Could you check a few things on this model? Use its own coordinates, in mm. Coordinates: 2 decimals unless noted, no trailing zeros. Write each loop counter-clockwise with the first axis right and the second up, starting at its lowest first coordinate (ties: lowest second). Pieces come first, ordered by that corner, then holes.
Item 1: If I drill on probe 1 along X at (y, z) = (66.5, 1.55); probe 2 along X at (y, z) = (56.5, 1.8); probe 3 along Y at (x, z) = (39, 1.8), over which ranges is the centre line in solid material (lowest first)?
Item 2: I want a section at A-A on x = 0. Please give me the cut outline in (y, z).
Item 3: I want a section at B-B on y = -71.5. Please give me the cut outline in (x, z), then the cut area to 3 significant figures.
Item 4: I want a section at D-D on y = 71.5. Please give me the cut outline in (x, z).
Item 5: I want a section at C-C on z = 1.2. State how many separate pieces and enclosed holes the cut face has, then the cut area to 3 significant figures.
Item 6: For P1, Ø1, axis at y = -6, z = 1, coming from the +X side, with a flat end and sliding along its axis, tell me the tip position at first contact or that it passes through.
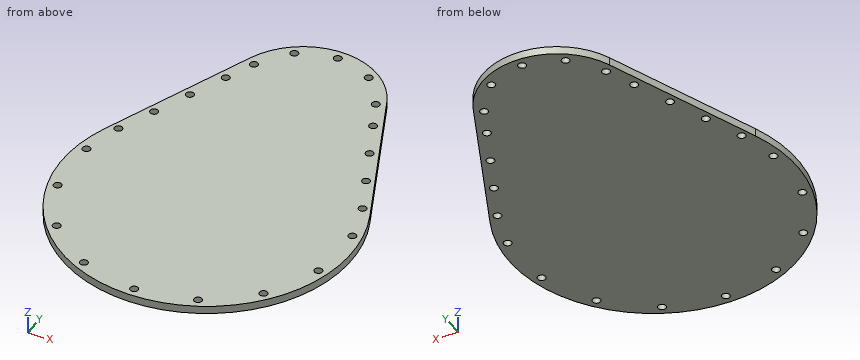
from build123d import *

# Parameters (mm, degrees)
SKETCH1_R           = 1.5
BOSS_EXTRUDE1_DEPTH = 3


with BuildPart() as part:
    # Sketch1 → Boss-Extrude1 (new body)
    with BuildSketch(Plane.XY):
        with BuildLine():
            Line((-25.751949598, 57.992592593), (-50.124330467, 0.896296296))
            ThreePointArc((-50.124330467, 0.896296296), (0, -75), (50.124330467, 0.896296296))
            Line((50.124330467, 0.896296296), (25.751949598, 57.992592593))
            ThreePointArc((25.751949598, 57.992592593), (0, 75), (-25.751949598, 57.992592593))
        make_face()
        with Locations((0, -71.5)):
            Circle(SKETCH1_R, mode=Mode.SUBTRACT)
        with Locations((0, 71.5)):
            Circle(SKETCH1_R, mode=Mode.SUBTRACT)
        with Locations((14.052622691, 67.069225085)):
            Circle(SKETCH1_R, mode=Mode.SUBTRACT)
        with Locations((23.022469209, 55.379493511)):
            Circle(SKETCH1_R, mode=Mode.SUBTRACT)
        with Locations((21.553531349, -66.721697139)):
            Circle(SKETCH1_R, mode=Mode.SUBTRACT)
        with Locations((39.068266599, -53.282168094)):
            Circle(SKETCH1_R, mode=Mode.SUBTRACT)
        with Locations((49.262217141, -33.6997713)):
            Circle(SKETCH1_R, mode=Mode.SUBTRACT)
        with Locations((50.225195404, -11.643942939)):
            Circle(SKETCH1_R, mode=Mode.SUBTRACT)
        with Locations((27.835315177, 44.555939465)):
            Circle(SKETCH1_R, mode=Mode.SUBTRACT)
        with Locations((33.935175216, 30.757307943)):
            Circle(SKETCH1_R, mode=Mode.SUBTRACT)
        with Locations((40.035035255, 16.95867642)):
            Circle(SKETCH1_R, mode=Mode.SUBTRACT)
        with Locations((46.134895294, 3.160044897)):
            Circle(SKETCH1_R, mode=Mode.SUBTRACT)
        with Locations((-46.134895294, 3.160044897)):
            Circle(SKETCH1_R, mode=Mode.SUBTRACT)
        with Locations((-40.035035255, 16.95867642)):
            Circle(SKETCH1_R, mode=Mode.SUBTRACT)
        with Locations((-33.935175216, 30.757307943)):
            Circle(SKETCH1_R, mode=Mode.SUBTRACT)
        with Locations((-27.835315177, 44.555939465)):
            Circle(SKETCH1_R, mode=Mode.SUBTRACT)
        with Locations((-50.225195404, -11.643942939)):
            Circle(SKETCH1_R, mode=Mode.SUBTRACT)
        with Locations((-49.262217141, -33.6997713)):
            Circle(SKETCH1_R, mode=Mode.SUBTRACT)
        with Locations((-39.068266599, -53.282168094)):
            Circle(SKETCH1_R, mode=Mode.SUBTRACT)
        with Locations((-21.553531349, -66.721697139)):
            Circle(SKETCH1_R, mode=Mode.SUBTRACT)
        with Locations((-23.022469209, 55.379493511)):
            Circle(SKETCH1_R, mode=Mode.SUBTRACT)
        with Locations((-14.052622691, 67.069225085)):
            Circle(SKETCH1_R, mode=Mode.SUBTRACT)
    extrude(amount=BOSS_EXTRUDE1_DEPTH)


solid = part.part
Response values:
1. probe 1: x = -20.09 to -15.44, -12.66 to 12.66, 15.44 to 20.09
1. probe 2: x = -26.39 to -24.02, -22.03 to 22.03, 24.02 to 26.39
1. probe 3: y = -58.57 to -54.78, -51.78 to 15.87, 18.04 to 26.96
2. outline: (-75, 0) - (-73, 0) - (-73, 3) - (-75, 3) - close; (-70, 0) - (70, 0) - (70, 3) - (-70, 3) - close; (73, 0) - (75, 0) - (75, 3) - (73, 3) - close
3. outline: (-19.22, 0) - (-1.5, 0) - (-1.5, 3) - (-19.22, 3) - close; (1.5, 0) - (19.22, 0) - (19.22, 3) - (1.5, 3) - close
3. area: 106 mm2
4. outline: (-13.56, 0) - (-1.5, 0) - (-1.5, 3) - (-13.56, 3) - close; (1.5, 0) - (13.56, 0) - (13.56, 3) - (1.5, 3) - close
5. separate pieces: 1
5. enclosed holes: 22
5. area: 11,700 mm2
6. P1: stops at x = 52.67
